Check sheet for the drawn part. Datum: minimum x, y, z corner. Units: mm. Coordinates: 2 decimals unless noted, no trailing zeros. Write each loop counter-clockwise with the first axis right and the second up, starting at its lowest first coordinate (ties: lowest second). Pieces come first, ordered by that corner, then holes. Notation, with made-up numbers: M 84.25,84.5 L 95.25,84.5 A14 cw 95.25,93.5 Z; hole C 80.25,-14.75 d10. An arc over 180 degrees is marked long. Write item = value, one per line. Start each with the question number.
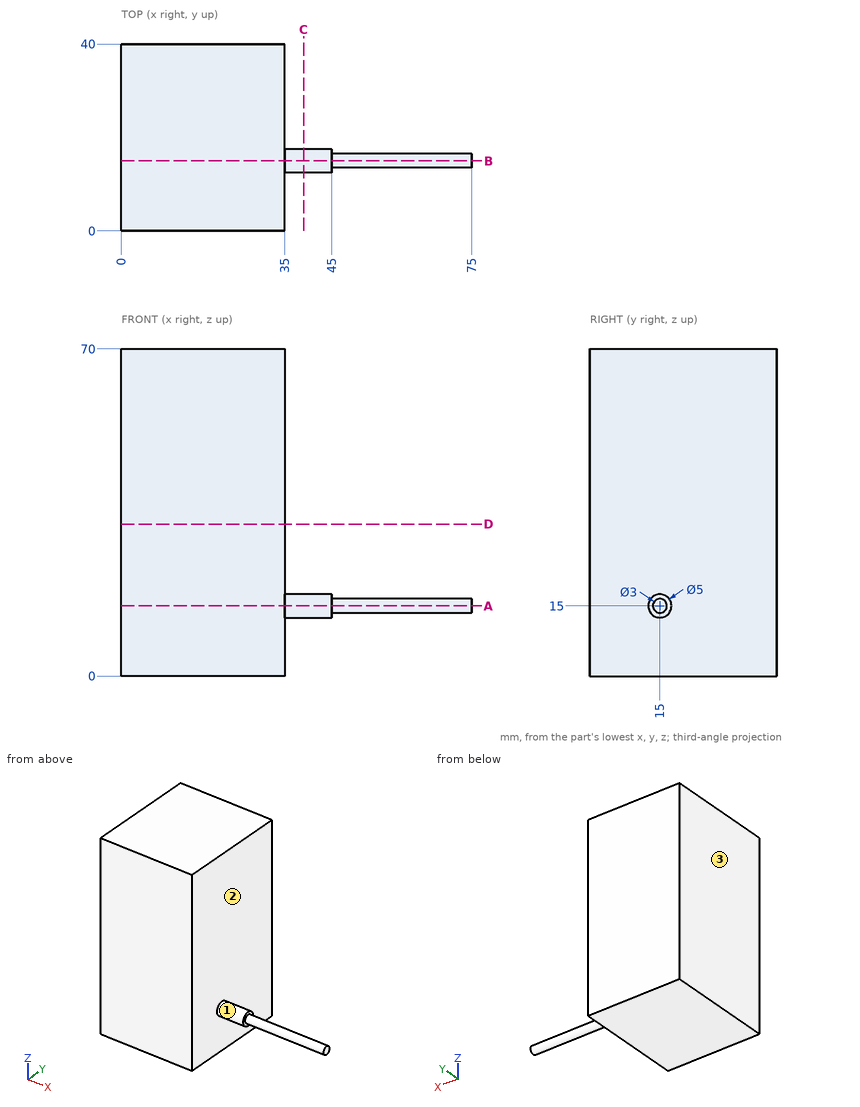
Q1. Gauge pin test, flat ends, axial feed: pin 1 (1.5 mm diameter, centred on x = 14, z = 50, fed in from -Y); pin 2 (10 mm diameter, centred on y = 22, z = 56.5, fed in from +X). Record the tip position at first contact, or that the pin passes through.
Q2. Cross-section at C-C on x = 39. Enter the section's corners in (y, z), and give its area (3 significant figures).
Q3. Cross-section at B-B on y = 15. Enter the section's corners in (x, z).
Q4. Draft check along X on the marked faces 1, 2 and 3. Enter one of: pulls with the +X half, pulls with the -X half, needs draft (parallel to the pull), parting line crosses it, or undercut.
Q5. Scan line: L1, parallel to X at y = 22, z = 4. Record every from-to range of solid material in increasing order.
Q6. Cross-section at A-A on z = 15. Enter the section's corners in (x, y), and give its area (3 significant figures).
Q7. Cross-section at D-D on z = 32.5. Enter the section's corners in (x, y).
Values found:
q1.pin_1 = 0
q1.pin_2 = 35
q2.outline = C 15,15 d5
q2.area = 19.6 mm²
q3.outline = M 0,0 L 35,0 L 35,12.5 L 45,12.5 L 45,13.5 L 75,13.5 L 75,16.5 L 45,16.5 L 45,17.5 L 35,17.5 L 35,70 L 0,70 Z
q4.face_1 = needs draft
q4.face_2 = pulls with the +X half
q4.face_3 = pulls with the -X half
q5.L1 = 0 to 35
q6.outline = M 0,0 L 35,0 L 35,12.5 L 45,12.5 L 45,13.5 L 75,13.5 L 75,16.5 L 45,16.5 L 45,17.5 L 35,17.5 L 35,40 L 0,40 Z
q6.area = 1,540 mm²
q7.outline = M 0,0 L 35,0 L 35,40 L 0,40 Z
